Read the model definition and answer for the solid it produces. Units are mm, in the model's axes. A direction names the side the tool comes from. Coordinates: 2 decimals unless noted, no trailing zeros. Write each loop counter-clockwise with the first axis right and the second up, starting at its lowest first coordinate (ties: lowest second). Pieces come first, ordered by that corner, then holes.
Item 1: Section A-A (x = -259) is taken. Give the vertices of the cut face in (y, z).
Item 2: Straight lines are drawn through the part: probe 1 along X at (y, z) = (-10, 228); probe 2 along X at (y, z) = (-60.5, 158); probe 3 along Z at (x, y) = (-285.5, -57.15). For each, find the intervals that lie inside material, in ascending order.
Item 3: Determine the mould class of faces 4 (the face through (386.36, -9.66, 7.24)), 5 (the face through (365, -38, 88.9)), 6 (the face through (336.851, -49.2, 144.5)) for opening direction X: released by +X, released by -X, zero draft, split by the parting line, or undercut.
Item 4: Section B-B (z = 136) is taken. Give the vertices of the cut face in (x, y).
Item 5: Each of these flat-tipped pins is pushed along its axis until it touches: P1, Ø5, axis at x = -229.5, z = 208, coming from the -Y side; P2, Ø11.5, axis at x = 359, y = -44.5, coming from the -Z side; P3, Ø19, axis at x = 378.5, y = -38.5, coming from the +Z side. Where does it stop, or does it pass through?
Item 6: Section D-D (x = 186) is taken. Give the vertices of the cut face in (y, z), then the cut area to 3 significant figures.
Item 7: Section C-C (z = 198.5) is taken. Give the vertices of the cut face in (x, y).
Item 8: A tool of negligible diameter and unlimited length cuts with its end or side. For faces 1 (the face through (365, -38, 165.1)), 2 (the face through (-247.349, -40, 136)), 3 (the face through (-276, -38, 88.9)), from which of +Z, -Z, +X, -X, +Y, -Y can it reach the whole face along a straight path? Write none if from no direction.
from build123d import *

# Parameters (mm, degrees)
F1_DEPTH  = 19.05
F2_R      = 25.4
F4_W      = 57.15
F4_H      = 38.1
F5_DEPTH  = 38.1
F7_DEPTH  = 57.15
F8_R      = 19.05
F10_DEPTH = 76.2
F12_DEPTH = 38.1
F14_DEPTH = 57.15
F16_DEPTH = 76.2
F15_R     = 19.05
F17_DEPTH = 57.15
F11_R     = 9.525
F18_DEPTH = 25.4


with BuildPart() as f1:
    # F0 (on Front) → F1 (new body)
    with BuildSketch(Plane.XZ):
        Polygon((-304.499298, 254), (-304.499298, 0), (44.750702, 0), (394.000702, 0), (394.000702, 254), align=None)
        with BuildLine():
            ThreePointArc((63.800702, 127), (58.221086, 113.529616), (44.750702, 107.95))
            ThreePointArc((44.750702, 107.95), (31.280317, 140.470384), (63.800702, 127))
        make_face(mode=Mode.SUBTRACT)
    extrude(amount=F1_DEPTH)

    # F2
    f2_edges = [f1.edges().sort_by_distance(p)[0] for p in [
        (-304.499298, -9.525, 254),
        (394.000702, -9.525, 254),
        (394.000702, -9.525, 0),
        (-304.499298, -9.525, 0),
    ]]
    fillet(f2_edges, radius=F2_R)

    # F4 (on face) → F5 (join)
    with BuildSketch(Plane.XZ.offset(19.05)):
        with Locations((-275.924298, 146.05)):
            Rectangle(F4_W, F4_H)
        with Locations((-275.924298, 107.95)):
            Rectangle(F4_W, F4_H)
    extrude(amount=F5_DEPTH)

    # F6 (on face) → F7 (join)
    with BuildSketch(Plane(origin=(-304.499298, 0, 0), x_dir=(0, -1, 0), z_dir=(-1, 0, 0))):
        with BuildLine():
            ThreePointArc((57.15, 88.9), (84.090768, 100.059232), (95.25, 127))
            ThreePointArc((95.25, 127), (84.090768, 153.940768), (57.15, 165.1))
            Line((57.15, 165.1), (57.15, 88.9))
        make_face()
    extrude(amount=-F7_DEPTH)

    # F8 (on face) → F10 (cut)
    with BuildSketch(Plane.YZ.offset(-247.349298)):
        with Locations((-57.15, 127)):
            Circle(F8_R)
    extrude(amount=-F10_DEPTH, mode=Mode.SUBTRACT)

    # F4 (on face) → F12 (join)
    with BuildSketch(Plane.XZ.offset(19.05)):
        with Locations((-275.924298, 146.05)):
            Rectangle(F4_W, F4_H)
        with Locations((-275.924298, 107.95)):
            Rectangle(F4_W, F4_H)
        with Locations((365.425702, 107.95)):
            Rectangle(F4_W, F4_H)
        with Locations((365.425702, 146.05)):
            Rectangle(F4_W, F4_H)
    extrude(amount=F12_DEPTH)

    # F13 (on face) → F14 (join)
    with BuildSketch(Plane.YZ.offset(394.000702)):
        with BuildLine():
            Line((-57.15, 88.9), (-57.15, 165.1))
            ThreePointArc((-57.15, 165.1), (-95.25, 127), (-57.15, 88.9))
        make_face()
    extrude(amount=-F14_DEPTH)

    # F8 (on face) → F16 (cut)
    with BuildSketch(Plane.YZ.offset(-247.349298)):
        with Locations((-57.15, 127)):
            Circle(F8_R)
    extrude(amount=-F16_DEPTH, mode=Mode.SUBTRACT)

    # F15 (on face) → F17 (cut)
    with BuildSketch(Plane.YZ.offset(394.000702)):
        with Locations((-57.15, 127)):
            Circle(F15_R)
    extrude(amount=-F17_DEPTH, mode=Mode.SUBTRACT)

    # F11 (on face) → F18 (cut)
    with BuildSketch(Plane.XZ.offset(19.05)):
        with Locations((-279.099298, 228.6)):
            Circle(F11_R)
        with Locations((-279.099298, 25.4)):
            Circle(F11_R)
        with Locations((368.600702, 228.6)):
            Circle(F11_R)
        with Locations((368.600702, 25.4)):
            Circle(F11_R)
    extrude(amount=-F18_DEPTH, mode=Mode.SUBTRACT)


solid = f1.part
Established:
1. outline: (-95.25, 127) arc R38.1 ccw to (-57.15, 88.9) - (-19.05, 88.9) - (-19.05, 0) - (0, 0) - (0, 254) - (-19.05, 254) - (-19.05, 165.1) - (-57.15, 165.1) arc R38.1 ccw to start; hole circle Ø38.1 at (-57.15, 127)
2. probe 1: x = -304.5 to -288.61, -269.59 to 359.09, 378.11 to 394
2. probe 2: x = -304.5 to -247.35, 336.85 to 394
2. probe 3: z = 88.9 to 107.95, 146.05 to 165.1
3. face 4: released by +X
3. face 5: zero draft
3. face 6: undercut
4. outline: (-304.5, -94.17) - (-247.35, -94.17) - (-247.35, -73.94) - (-304.5, -73.94) - close; (-304.5, -40.36) - (-247.35, -40.36) - (-247.35, -19.05) - (27.96, -19.05) - (27.96, 0) - (-304.5, 0) - close; (61.54, -19.05) - (336.85, -19.05) - (336.85, -40.36) - (394, -40.36) - (394, 0) - (61.54, 0) - close; (336.85, -94.17) - (394, -94.17) - (394, -73.94) - (336.85, -73.94) - close
5. P1: stops at y = -19.05
5. P2: stops at z = 88.9
5. P3: stops at z = 165.1
6. outline: (-19.05, 0) - (0, 0) - (0, 254) - (-19.05, 254) - close
6. area: 4,840 mm2
7. outline: (-304.5, -19.05) - (394, -19.05) - (394, 0) - (-304.5, 0) - close
8. face 1: +Z, +X, -X, -Y
8. face 2: +Z, -Z, -Y
8. face 3: -Z, +X, -X, -Y
